Check sheet for the modelled part. Datum: model origin and axes. Units: mm. Face numbers are marked on the shaded views. A direction names the side the tool comes from. Round coordinates to 2 decimals unless told otherwise and drop trailing zeros. Write each loop counter-clockwise with the first axis right and the second up, starting at its lowest first coordinate (ties: lowest second). Pieces come first, ordered by that corner, then holes. Notation, with made-up numbers: (-8, 17.25) - (13, 17.25) arc R26 cw to (13, 35.25) - close; hole circle Ø8 at (71.5, -26). An arc over 180 degrees is marked (long way). Use one line per item in the form item = value. Start each with the question number.
1) Section check A-A (y = 2.25). Record the boundary of the cut face in (x, z).
2) Section check C-C (x = 2.5). Record the boundary of the cut face in (y, z), then the cut area to 3 significant figures.
3) Scan lines: probe 1 along X at (y, z) = (6.5, -4); probe 2 along Z at (x, y) = (28, 18). Record each from-to range of solid material in increasing order.
4) Section check B-B (z = 13). Record the boundary of the cut face in (x, y).
5) Gauge pin test, flat end, axial feed: P1, Ø5, axis at x = -11.5, z = -29.5, coming from the -Y side. Record the tip position at first contact, or that the pin passes through.
6) Draft check along Z on the marked faces 1, 2 and 3. Enter one of: +Z half, -Z half, draft (parallel to the pull), parting line (faces both ways), or undercut.
7) Set-up check for the marked faces 4 and 5: record each of +Z, -Z, +X, -X, +Y, -Y from which the full face is reachable in a straight line by a thin tool's end or side.
8) Section check D-D (y = 12.7). Count the separate pieces of the cut face and the enclosed holes in it, then the cut area to 3 significant figures.
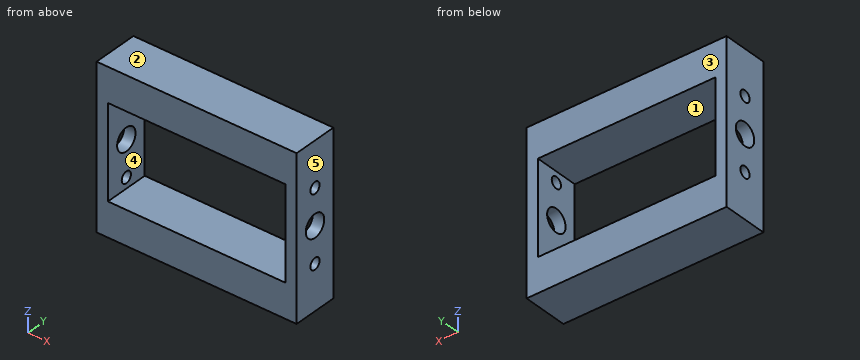
from build123d import *

# Parameters (mm, degrees)
CROQUIS1_W              = 150.1
CROQUIS1_H              = 90
CROQUIS1_W_2            = 99.3
CROQUIS1_H_2            = 51.9
SALIENTE_EXTRUIR1_DEPTH = 25.4
CROQUIS2_R              = 6.35
SALIENTE_EXTRUIR2_DEPTH = 51.85
SALIENTE_EXTRUIR3_START = -174.15
CROQUIS2_2_R            = 6.35
SALIENTE_EXTRUIR3_DEPTH = 24.05
CROQUIS4_R              = 3.175
CORTAR_EXTRUIR2_DEPTH   = 182.654569169
CORTAR_EXTRUIR3_START   = 51.85
CROQUIS2_3_R            = 6.35
CORTAR_EXTRUIR3_DEPTH   = 234.504569169
CROQUIS6_W              = 19.05
CROQUIS6_H              = 90
CORTAR_EXTRUIR4_DEPTH   = 92.118946987


with BuildPart() as part:
    # Croquis1 → Saliente-Extruir1 (new body)
    with BuildSketch(Plane(origin=(0, 0, 0), x_dir=(1, 0, 0), z_dir=(0, 1, 0))):
        Rectangle(CROQUIS1_W, CROQUIS1_H)
        Rectangle(CROQUIS1_W_2, CROQUIS1_H_2, mode=Mode.SUBTRACT)
    extrude(amount=SALIENTE_EXTRUIR1_DEPTH)

    # Croquis2 → Saliente-Extruir2 (add)
    with BuildSketch(Plane(origin=(75.05, 0, 0), x_dir=(0, 0, -1), z_dir=(1, 0, 0))):
        with Locations(Location((0, 12.7, 0), (0, 0, 180))):
            Circle(CROQUIS2_R)
    extrude(amount=SALIENTE_EXTRUIR2_DEPTH)

    # Croquis2<2> → Saliente-Extruir3 (add)
    with BuildSketch(Plane(origin=(75.05, 0, 0), x_dir=(0, 0, -1), z_dir=(1, 0, 0)).offset(SALIENTE_EXTRUIR3_START)):
        with Locations(Location((0, 12.7, 0), (0, 0, 180))):
            Circle(CROQUIS2_2_R)
    extrude(amount=SALIENTE_EXTRUIR3_DEPTH)

    # Croquis4 → Cortar-Extruir2 (cut, through all)
    with BuildSketch(Plane(origin=(75.05, 0, 0), x_dir=(0, 0, -1), z_dir=(1, 0, 0))):
        with Locations((-20, 12.7)):
            Circle(CROQUIS4_R)
        with Locations((20, 12.7)):
            Circle(CROQUIS4_R)
    extrude(amount=-CORTAR_EXTRUIR2_DEPTH, mode=Mode.SUBTRACT)

    # Croquis2<3> → Cortar-Extruir3 (cut, through all)
    with BuildSketch(Plane(origin=(75.05, 0, 0), x_dir=(0, 0, -1), z_dir=(1, 0, 0)).offset(CORTAR_EXTRUIR3_START)):
        with Locations(Location((0, 12.7, 0), (0, 0, 180))):
            Circle(CROQUIS2_3_R)
    extrude(amount=-CORTAR_EXTRUIR3_DEPTH, mode=Mode.SUBTRACT)

    # Croquis6 → Cortar-Extruir4 (cut, through all)
    with BuildSketch(Plane(origin=(0, 25.4, 0), x_dir=(1, 0, 0), z_dir=(0, 1, 0))):
        with Locations((-65.525, 0)):
            Rectangle(CROQUIS6_W, CROQUIS6_H)
        with Locations((65.525, 0)):
            Rectangle(CROQUIS6_W, CROQUIS6_H)
    extrude(amount=-CORTAR_EXTRUIR4_DEPTH, mode=Mode.SUBTRACT)


solid = part.part
Results are:
q1.outline = (-56, -45) - (56, -45) - (56, 45) - (-56, 45) - close; hole (-49.65, -25.95) - (49.65, -25.95) - (49.65, 25.95) - (-49.65, 25.95) - close
q2.outline = (0, -45) - (25.4, -45) - (25.4, -25.95) - (0, -25.95) - close; (0, 25.95) - (25.4, 25.95) - (25.4, 45) - (0, 45) - close
q2.area = 968 mm²
q3.probe_1 = -56 to -49.65, 49.65 to 56
q3.probe_2 = -45 to -25.95, 25.95 to 45
q4.outline = (-56, 0) - (-49.65, 0) - (-49.65, 25.4) - (-56, 25.4) - close; (49.65, 0) - (56, 0) - (56, 25.4) - (49.65, 25.4) - close
q5.P1 = 0
q6.face_1 = undercut
q6.face_2 = +Z half
q6.face_3 = draft
q7.face_4 = +Y, -Y
q7.face_5 = +Z, -Z, +X, +Y, -Y
q8.separate_pieces = 6
q8.enclosed_holes = 0
q8.area = 4,600 mm²
